Geometry: final body of the model. Coordinates: model frame, mm. A direction names the side the tool comes from. Round coordinates to 2 decimals unless told otherwise and drop trailing zeros. Write each loop counter-clockwise with the first axis right and the second up, starting at its lowest first coordinate (ties: lowest second). Pieces come first, ordered by that corner, then holes. Notation, with made-up numbers: (69, -21.5) - (79, -21.5) arc R11 cw to (79, -17.5) - close; hole circle Ø8 at (37, 54.5). An arc over 180 degrees is marked (long way). Write each question's results on one line, items separated by ' | '.
from build123d import *

# Parameters (mm, degrees)
BOSS_EXTRUDE3_DEPTH = 10.82
BOSS_EXTRUDE4_DEPTH = 3.9
SKETCH3_R           = 1
CUT_EXTRUDE1_DEPTH  = 5.25
CUT_EXTRUDE2_DEPTH  = 10


with BuildPart() as part:
    # Sketch2 → Boss-Extrude3 (new body)
    with BuildSketch(Plane.XY):
        Polygon((8.44, 0), (3, 0), (1.25, 0), (1.25, -5.25), (3, -5.25), (8.44, -5.25), align=None)
    extrude(amount=BOSS_EXTRUDE3_DEPTH)

    # Sketch2<5> → Boss-Extrude4 (add)
    with BuildSketch(Plane.XY):
        with BuildLine():
            Line((31.5, 0), (8.44, 0))
            Line((8.44, 0), (8.44, -5.25))
            ThreePointArc((8.44, -5.25), (12.24, -6.85540936), (16.04, -5.25))
            Line((16.04, -5.25), (31.5, -5.25))
            Line((31.5, -5.25), (31.5, 0))
        make_face()
    extrude(amount=BOSS_EXTRUDE4_DEPTH)

    # Sketch3 → Cut-Extrude1 (cut)
    with BuildSketch(Plane(origin=(0, 0, 0), x_dir=(1, 0, 0), z_dir=(0, 1, 0))):
        with Locations(Location((4.845, -2.5, 0), (0, 0, 270))):
            Circle(SKETCH3_R)
        with Locations(Location((4.845, -8, 0), (0, 0, 270))):
            Circle(SKETCH3_R)
    extrude(amount=-CUT_EXTRUDE1_DEPTH, mode=Mode.SUBTRACT)

    # Sketch4 → Cut-Extrude2 (cut)
    with BuildSketch(Plane(origin=(0, 0, 0), x_dir=(1, 0, 0), z_dir=(0, 1, 0))):
        Polygon((1.25, 0), (1.25, -0.249924402), (31.493852375, -0.249924402), (31.5, 0), align=None)
    extrude(amount=-CUT_EXTRUDE2_DEPTH, mode=Mode.SUBTRACT)


solid = part.part
Q1. Ray query, line 1 along X through (y, z) = (-2.85, 8) (3 decimals); line 2 along Z through (x, y) = (3, -3); line 3 along X through (y, z) = (-3.5, 2.5) (3 decimals). Return the intervals inside material, ascending.
Answer block:
line 1: 1.25 to 3.845, 5.845 to 8.44 | line 2: 0.25 to 10.82 | line 3: 1.25 to 3.845, 5.845 to 31.5
Q2. Mould query, pull axis X, two halves, no side actions, for faces 1 (the cylindrical face through (12.181, -6.855, 2.049)), 2 (the cylindrical face through (5.52, -2.59, 1.76)), 3 (the flat face through (16, -3, 0.25)). Classes: pulls with the +X half, pulls with the -X half, needs draft (parallel to the pull), parting line crosses it, or undercut.
Answer block:
face 1: parting line crosses it | face 2: undercut | face 3: needs draft
Q3. Access query for faces 4 (the flat face through (20, -3, 3.9)), 5 (the flat face through (5, -5.25, 5)), 6 (the flat face through (24, -5.25, 2)). Directions: +Z, -Z, +X, -X, +Y, -Y. A direction counts if a zero-diameter tool reaches every point of the face in a straight line with its end or side. Return the directions, or none.
Answer block:
face 4: +Z, +X, +Y, -Y | face 5: +Z, -Z, -X, -Y | face 6: +Z, -Z, +X, -Y
Q4. Pin query (flat end, axial travel): pin 1 (1.5 mm diameter, centred on x = 20.5, y = -1, fed in from +Z); pin 2 (2.5 mm diameter, centred on x = 4.845, z = 2.5, fed in from +Y); pin 3 (2 mm diameter, centred on x = 15.5, z = 2, fed in from -Y); pin 4 (2 mm diameter, centred on x = 26.5, z = 1.5, fed in from -Y). Return the tip coordinate at first contact, or that it passes through.
Answer block:
pin 1: z = 3.9 | pin 2: y = 0 | pin 3: y = -6.35 | pin 4: y = -5.25
Q5. Section query A-A, the plane z = 8. Return loops of the section in (x, y) (3 decimals).
Answer block:
outline: (1.25, -5.25) - (3.845, -5.25) - (3.845, 0) - (1.25, 0) - close; (5.845, -5.25) - (8.44, -5.25) - (8.44, 0) - (5.845, 0) - close
Q6. Section query B-B, the plane x = 20. Return loops of the section in (y, z).
Answer block:
outline: (-5.25, 0.25) - (0, 0.25) - (0, 3.9) - (-5.25, 3.9) - close
Q7. Section query D-D, the plane y = -3. Return loops of the section in (x, z) (3 decimals).
Answer block:
outline: (1.25, 0.25) - (31.494, 0.25) - (31.5, 0) - (31.5, 3.9) - (8.44, 3.9) - (8.44, 10.82) - (1.25, 10.82) - close; hole circle Ø2 at (4.845, 2.5); hole circle Ø2 at (4.845, 8)
Q8. Section query C-C, the plane z = 2.5. Return loops of the section in (x, y) (3 decimals).
Answer block:
outline: (1.25, -5.25) - (3.845, -5.25) - (3.845, 0) - (1.25, 0) - close; (5.845, -5.25) - (8.44, -5.25) arc R5.3 ccw to (16.04, -5.25) - (31.5, -5.25) - (31.5, 0) - (5.845, 0) - close
